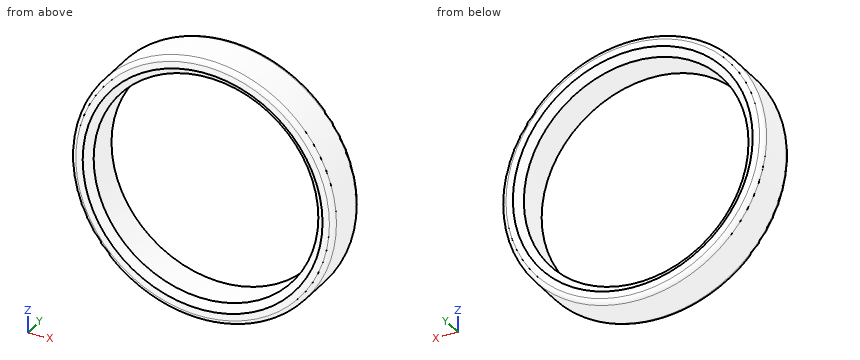
```python
from build123d import *

# Parameters (mm, degrees)
F3_R = 2
F4_R = 2


with BuildPart() as f2:
    # F0 (on Top) → F2 (revolve)
    with BuildSketch(Plane.XY):
        Polygon((52.305677, 10), (49, 7.25), (49, -7.25), (52.305677, -10), (57.305677, -10), (57.305677, 10), align=None)
    revolve(axis=Axis((0, -6.822679, 0), (0, 1, 0)))

    # F3
    f3_edges = [f2.edges().sort_by_distance(p)[0] for p in [
        (-57.305677, -10, 0),
    ]]
    fillet(f3_edges, radius=F3_R)

    # F4
    f4_edges = [f2.edges().sort_by_distance(p)[0] for p in [
        (-57.305677, 10, 0),
    ]]
    fillet(f4_edges, radius=F4_R)


solid = f2.part
```
Work out the finished part from the listing and answer in its coordinate system (mm). Round coordinates to 2 decimals unless told otherwise and drop trailing zeros. Write each loop counter-clockwise with the first axis right and the second up, starting at its lowest first coordinate (ties: lowest second). Pieces come first, ordered by that corner, then holes.
1) Flat-ended cylindrical pins translate along their axes: P1, Ø8, axis at x = 43.5, y = 6, coming from the +Z side; P2, Ø4, axis at y = 6, z = 22.5, coming from the +X side; P3, Ø1, axis at x = -1.5, y = -2, coming from the -Z side. Find the tip coordinate at first contact, or state that the pin passes through.
2) A cutting plane is placed at B-B on z = 0. Determine the outline of the cut face in (x, y), and give its area (3 significant figures).
3) A cutting plane is placed at C-C on y = -5. Determine the outline of the cut face in (x, z).
4) Consider probe 1 along X at (y, z) = (-0.5, 0); probe 2 along Z at (x, y) = (29.5, -1.5). Determine where each line is inside the solid, lowest interval first.
5) A cutting plane is placed at A-A on x = 0. Determine the outline of the cut face in (y, z), and give its area (3 significant figures).
Entries:
1. P1: stops at z = 41.52
1. P2: stops at x = 53.51
1. P3: stops at z = -57.3
2. outline: (-57.31, -8) arc R2 ccw to (-55.31, -10) - (-52.31, -10) - (-49, -7.25) - (-49, 7.25) - (-52.31, 10) - (-55.31, 10) arc R2 ccw to (-57.31, 8) - close; (49, -7.25) - (52.31, -10) - (55.31, -10) arc R2 ccw to (57.31, -8) - (57.31, 8) arc R2 ccw to (55.31, 10) - (52.31, 10) - (49, 7.25) - close
2. area: 311 mm2
3. outline: circle Ø114.61 at (0, 0); hole circle Ø98 at (0, 0)
4. probe 1: x = -57.31 to -49, 49 to 57.31
4. probe 2: z = -49.13 to -39.12, 39.12 to 49.13
5. outline: (-10, -55.31) arc R2 ccw to (-8, -57.31) - (8, -57.31) arc R2 ccw to (10, -55.31) - (10, -52.31) - (7.25, -49) - (-7.25, -49) - (-10, -52.31) - close; (-10, 52.31) - (-7.25, 49) - (7.25, 49) - (10, 52.31) - (10, 55.31) arc R2 ccw to (8, 57.31) - (-8, 57.31) arc R2 ccw to (-10, 55.31) - close
5. area: 311 mm2
